Part print with two shaded views. Sizes in mm from the minimum x, y, z corner. Give positions to 0.01 mm unless a question says otherwise; leave off trailing zeros. Order: outer loops, then holes, each group sorted by start corner. A loop starts at its lowest first (then second) coordinate and runs counter-clockwise, first axis right, second up. Notation, with made-up numbers: (89, -29.75) - (111, -29.75) arc R25 cw to (111, -8.75) - close; hole circle Ø11 at (57.5, -4). An arc over 180 degrees is marked (long way). Return JSON: item names as keys, results as strings. Group by question number.
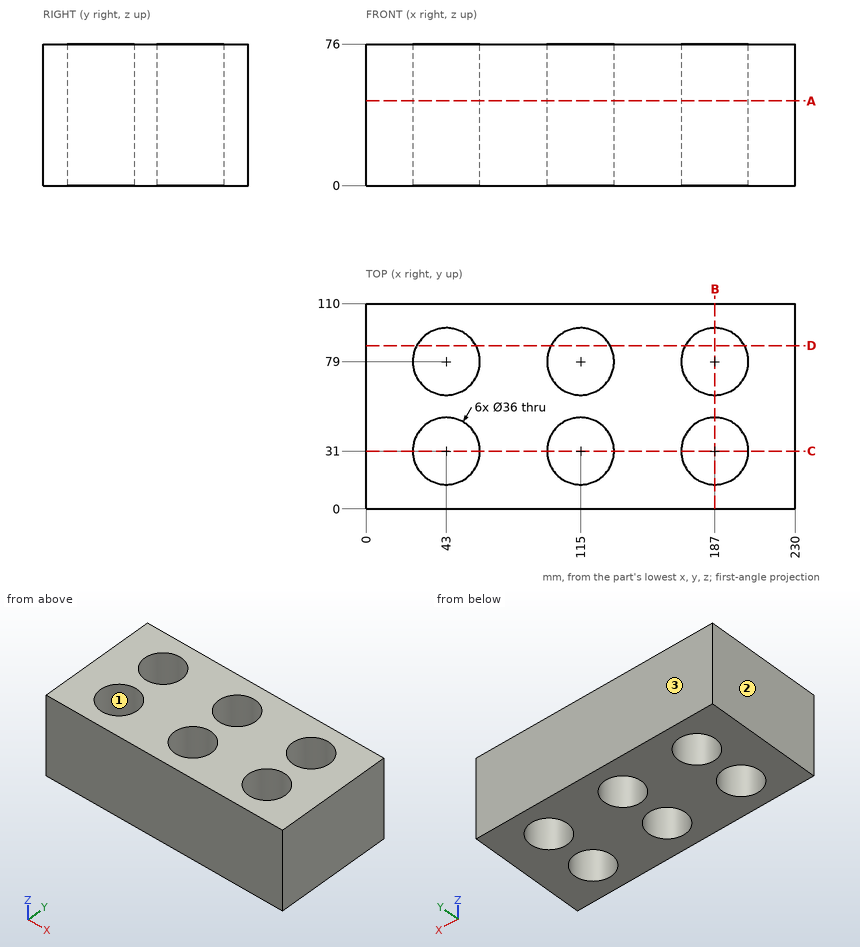
(1) Slice it at B-B (x = 187). Give the cut face in (y, z).
(2) Slice it at C-C (y = 31). Give the cut face in (x, z), and give its area (3 significant figures).
(3) Slice it at A-A (z = 45.5). Give the cut face in (x, y), and give its area (3 significant figures).
(4) Drill centre lines: L1, parallel to Y at x = 115, z = 35; L2, parallel to Y at x = 57, z = 44; L3, parallel to X at y = 45.5, z = 31.5. Where is each one in solid material? Low to high.
(5) Pull direction Y, two halves, no side cores. Call the marked faces 1, 2 and 3: released by +Y, released by -Y, zero draft, split by the parting line, or undercut.
(6) Slice it at D-D (y = 87.5). Give the cut face in (x, z), and give its area (3 significant figures).
(7) Drop a flat-ended pin along its axis: pin 1 Ø3 at (x, z) = (76.5, 68) entering from -Y. Give the stop position or say it passes through.
Result set:
{
 "1": {"outline": "(0, 0) - (13, 0) - (13, 76) - (0, 76) - close; (49, 0) - (61, 0) - (61, 76) - (49, 76) - close; (97, 0) - (110, 0) - (110, 76) - (97, 76) - close"},
 "2": {"outline": "(0, 0) - (25, 0) - (25, 76) - (0, 76) - close; (61, 0) - (97, 0) - (97, 76) - (61, 76) - close; (133, 0) - (169, 0) - (169, 76) - (133, 76) - close; (205, 0) - (230, 0) - (230, 76) - (205, 76) - close", "area": "9,270 mm²"},
 "3": {"outline": "(0, 0) - (230, 0) - (230, 110) - (0, 110) - close; hole circle Ø36 at (43, 31); hole circle Ø36 at (43, 79); hole circle Ø36 at (115, 31); hole circle Ø36 at (115, 79); hole circle Ø36 at (187, 31); hole circle Ø36 at (187, 79)", "area": "19,200 mm²"},
 "4": {"L1": "y = 0 to 13, 49 to 61, 97 to 110", "L2": "y = 0 to 19.69, 42.31 to 67.69, 90.31 to 110", "L3": "x = 0 to 32.33, 53.67 to 104.33, 125.67 to 176.33, 197.67 to 230"},
 "5": {"face 1": "undercut", "face 2": "zero draft", "face 3": "released by +Y"},
 "6": {"outline": "(0, 0) - (27.13, 0) - (27.13, 76) - (0, 76) - close; (58.87, 0) - (99.13, 0) - (99.13, 76) - (58.87, 76) - close; (130.87, 0) - (171.13, 0) - (171.13, 76) - (130.87, 76) - close; (202.87, 0) - (230, 0) - (230, 76) - (202.87, 76) - close", "area": "10,200 mm²"},
 "7": {"pin 1": "stops at y = 0"}
}
